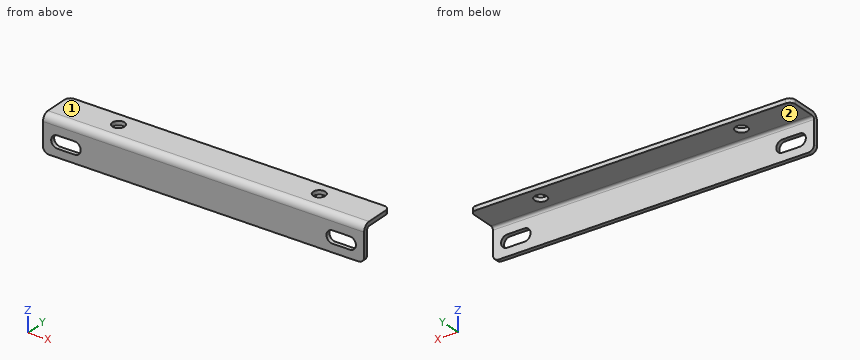
```python
from build123d import *

# Parameters (mm, degrees)
EXTRUDE1_DEPTH             = 88.9
FILLET1_R                  = 3.18
EXTRUDE2_REACH             = 94.271
EXTRUDE3_REACH             = 93.995
SKETCH3_R                  = 3.4036
FLATTEN_BENDS1_START       = -1.524
FLATTEN_BENDS1_OUTLINE_W   = 177.8
FLATTEN_BENDS1_OUTLINE_H   = 5.286
FLATTEN_BENDS1_DEPTH       = 17.4498
FLATTEN_BENDS1_START_2     = -3.81
FLATTEN_BENDS1_2_OUTLINE_R = 3.4036
FLATTEN_BENDS1_2_DEPTH     = 2.286
PROCESS_BENDS1_START       = 2.234903703
PROCESS_BENDS1_OUTLINE_W   = 177.8
PROCESS_BENDS1_OUTLINE_H   = 2.286
PROCESS_BENDS1_DEPTH       = 16.356210101
PROCESS_BENDS1_2_OUTLINE_R = 3.4036
PROCESS_BENDS1_2_DEPTH     = 1.8835878
PROCESS_BENDS1_START_2     = 2.04455268
PROCESS_BENDS1_3_OUTLINE_W = 177.8
PROCESS_BENDS1_3_OUTLINE_H = 2.286
PROCESS_BENDS1_3_DEPTH     = 0.190351023
PROCESS_BENDS1_START_3     = -1.524
PROCESS_BENDS1_4_OUTLINE_R = 3.4036
PROCESS_BENDS1_4_DEPTH     = 3.81
PROCESS_BENDS1_START_4     = -88.9
PROCESS_BENDS1_5_DEPTH     = 177.8


with BuildPart() as part:
    # Sketch1 → Extrude1 (new, symmetric)
    with BuildSketch(Plane(origin=(0, 0, 0), x_dir=(0, 0, -1), z_dir=(1, 0, 0))):
        with BuildLine():
            Line((17.5006, -3.81), (17.5006, -1.524))
            Line((17.5006, -1.524), (1.524, -1.524))
            ThreePointArc((1.524, -1.524), (0.446369265, -1.077630735), (0, 0))
            Line((0, 0), (0, 15.9258))
            Line((0, 15.9258), (-2.286, 15.9258))
            Line((-2.286, 15.9258), (-2.286, 0))
            ThreePointArc((-2.286, 0), (-1.170076836, -2.694076836), (1.524, -3.81))
            Line((1.524, -3.81), (17.5006, -3.81))
        make_face()
    extrude(amount=EXTRUDE1_DEPTH, both=True)

    # Fillet1
    fillet1_edges = [part.edges().sort_by_distance(p)[0] for p in [
        (-88.9, -2.667, -17.5006),
        (88.9, 15.9258, 1.143),
        (88.9, -2.667, -17.5006),
        (-88.9, 15.9258, 1.143),
    ]]
    fillet(fillet1_edges, radius=FILLET1_R)

    # Sketch2 → Extrude2 (cut, up to next)
    with BuildSketch(Plane(origin=(0, -1.524, 0), x_dir=(1, 0, 0), z_dir=(0, 1, 0)), mode=Mode.PRIVATE) as extrude2_sk1:
        with BuildLine():
            Line((80.9625, 12.9667), (71.4375, 12.9667))
            ThreePointArc((71.4375, 12.9667), (68.0339, 9.5631), (71.4375, 6.1595))
            Line((71.4375, 6.1595), (80.9625, 6.1595))
            ThreePointArc((80.9625, 6.1595), (84.3661, 9.5631), (80.9625, 12.9667))
        make_face()
    extrude2_tool1 = extrude(extrude2_sk1.sketch, amount=-EXTRUDE2_REACH, mode=Mode.PRIVATE) & part.part
    # Sketch2 → Extrude2 (cut, up to next)
    with BuildSketch(Plane(origin=(0, -1.524, 0), x_dir=(1, 0, 0), z_dir=(0, 1, 0)), mode=Mode.PRIVATE) as extrude2_sk2:
        with BuildLine():
            Line((-71.4375, 6.1595), (-80.9625, 6.1595))
            ThreePointArc((-80.9625, 6.1595), (-84.3661, 9.5631), (-80.9625, 12.9667))
            Line((-80.9625, 12.9667), (-71.4375, 12.9667))
            ThreePointArc((-71.4375, 12.9667), (-68.0339, 9.5631), (-71.4375, 6.1595))
        make_face()
    extrude2_tool2 = extrude(extrude2_sk2.sketch, amount=-EXTRUDE2_REACH, mode=Mode.PRIVATE) & part.part
    add(extrude2_tool1.solids().sort_by_distance((76.2, -1.524, -9.5631))[0], mode=Mode.SUBTRACT)
    add(extrude2_tool2.solids().sort_by_distance((-76.2, -1.524, -9.5631))[0], mode=Mode.SUBTRACT)

    # Sketch3 → Extrude3 (cut, up to next)
    with BuildSketch(Plane(origin=(0, 0, 0), x_dir=(-1, 0, 0), z_dir=(0, 0, -1)), mode=Mode.PRIVATE) as extrude3_sk1:
        with Locations(Location((-55.5625, 8.001, 0), (0, 0, 90))):
            Circle(SKETCH3_R)
    extrude3_tool1 = extrude(extrude3_sk1.sketch, amount=-EXTRUDE3_REACH, mode=Mode.PRIVATE) & part.part
    # Sketch3 → Extrude3 (cut, up to next)
    with BuildSketch(Plane(origin=(0, 0, 0), x_dir=(-1, 0, 0), z_dir=(0, 0, -1)), mode=Mode.PRIVATE) as extrude3_sk2:
        with Locations(Location((55.5625, 8.001, 0), (0, 0, 90))):
            Circle(SKETCH3_R)
    extrude3_tool2 = extrude(extrude3_sk2.sketch, amount=-EXTRUDE3_REACH, mode=Mode.PRIVATE) & part.part
    add(extrude3_tool1.solids().sort_by_distance((55.5625, 8.001, 0))[0], mode=Mode.SUBTRACT)
    add(extrude3_tool2.solids().sort_by_distance((-55.5625, 8.001, 0))[0], mode=Mode.SUBTRACT)

    # Flatten-Bends1: read off the stored shape, not the designer's step
    # Flatten-Bends1 outline → Flatten-Bends1 (cut)
    with BuildSketch(Plane(origin=(0, 0, 0), x_dir=(1, 0, 0), z_dir=(0, 1, 0)).offset(FLATTEN_BENDS1_START)):
        with Locations((0, 0.357)):
            Rectangle(FLATTEN_BENDS1_OUTLINE_W, FLATTEN_BENDS1_OUTLINE_H)
    extrude(amount=FLATTEN_BENDS1_DEPTH, mode=Mode.SUBTRACT)

    # Flatten-Bends1 2 outline → Flatten-Bends1 2 (add)
    with BuildSketch(Plane(origin=(0, 0, 0), x_dir=(1, 0, 0), z_dir=(0, 1, 0)).offset(FLATTEN_BENDS1_START_2)):
        with BuildLine():
            ThreePointArc((-88.9, -15.411113804), (-87.968599564, -17.659713368), (-85.72, -18.591113804))
            Line((-85.72, -18.591113804), (85.72, -18.591113804))
            ThreePointArc((85.72, -18.591113804), (87.968599564, -17.659713368), (88.9, -15.411113804))
            Line((88.9, -15.411113804), (88.9, 3))
            Line((88.9, 3), (-88.9, 3))
            Line((-88.9, 3), (-88.9, -15.411113804))
        make_face()
        with Locations((-55.5625, -10.666313804)):
            Circle(FLATTEN_BENDS1_2_OUTLINE_R, mode=Mode.SUBTRACT)
        with Locations((55.5625, -10.666313804)):
            Circle(FLATTEN_BENDS1_2_OUTLINE_R, mode=Mode.SUBTRACT)
    extrude(amount=FLATTEN_BENDS1_2_DEPTH)

    # Process-Bends1: read off the stored shape, not the designer's step
    # Process-Bends1 outline → Process-Bends1 (cut)
    with BuildSketch(Plane.XY.offset(PROCESS_BENDS1_START)):
        with Locations((0, -2.667)):
            Rectangle(PROCESS_BENDS1_OUTLINE_W, PROCESS_BENDS1_OUTLINE_H)
    extrude(amount=PROCESS_BENDS1_DEPTH, mode=Mode.SUBTRACT)

    # Process-Bends1 2 outline → Process-Bends1 2 (add)
    with BuildSketch(Plane.XY):
        with BuildLine():
            Line((-88.9, 12.7458), (-88.9, -1.524))
            Line((-88.9, -1.524), (88.9, -1.524))
            Line((88.9, -1.524), (88.9, 12.7458))
            ThreePointArc((88.9, 12.7458), (87.968599564, 14.994399564), (85.72, 15.9258))
            Line((85.72, 15.9258), (-85.72, 15.9258))
            ThreePointArc((-85.72, 15.9258), (-87.968599564, 14.994399564), (-88.9, 12.7458))
        make_face()
        with Locations((-55.5625, 8.001)):
            Circle(PROCESS_BENDS1_2_OUTLINE_R, mode=Mode.SUBTRACT)
        with Locations((55.5625, 8.001)):
            Circle(PROCESS_BENDS1_2_OUTLINE_R, mode=Mode.SUBTRACT)
    extrude(amount=PROCESS_BENDS1_2_DEPTH)

    # Process-Bends1 3 outline → Process-Bends1 3 (cut)
    with BuildSketch(Plane.XY.offset(PROCESS_BENDS1_START_2)):
        with Locations((0, -2.667)):
            Rectangle(PROCESS_BENDS1_3_OUTLINE_W, PROCESS_BENDS1_3_OUTLINE_H)
    extrude(amount=PROCESS_BENDS1_3_DEPTH, mode=Mode.SUBTRACT)

    # Process-Bends1 4 outline → Process-Bends1 4 (add)
    with BuildSketch(Plane.XY.offset(PROCESS_BENDS1_START_3)):
        with BuildLine():
            Line((-88.9, 12.7458), (-88.9, -1.524))
            Line((-88.9, -1.524), (88.9, -1.524))
            Line((88.9, -1.524), (88.9, 12.7458))
            ThreePointArc((88.9, 12.7458), (87.968599564, 14.994399564), (85.72, 15.9258))
            Line((85.72, 15.9258), (-85.72, 15.9258))
            ThreePointArc((-85.72, 15.9258), (-87.968599564, 14.994399564), (-88.9, 12.7458))
        make_face()
        with Locations((-55.5625, 8.001)):
            Circle(PROCESS_BENDS1_4_OUTLINE_R, mode=Mode.SUBTRACT)
        with Locations((55.5625, 8.001)):
            Circle(PROCESS_BENDS1_4_OUTLINE_R, mode=Mode.SUBTRACT)
    extrude(amount=PROCESS_BENDS1_4_DEPTH)

    # Process-Bends1 5 outline → Process-Bends1 5 (cut)
    with BuildSketch(Plane.YZ.offset(PROCESS_BENDS1_START_4)):
        with BuildLine():
            Line((15.9258, -1.524), (15.9258, 0))
            Line((15.9258, 0), (0, 0))
            ThreePointArc((0, 0), (-1.077630735, -0.446369265), (-1.524, -1.524))
            Line((-1.524, -1.524), (15.9258, -1.524))
        make_face()
        with BuildLine():
            ThreePointArc((-3.81, -1.524), (-2.694076836, 1.170076836), (0, 2.286))
            Line((0, 2.286), (-1.524, 2.286))
            Line((-1.524, 2.286), (-1.524, 2.04455268))
            Line((-1.524, 2.04455268), (-3.81, 2.04455268))
            Line((-3.81, 2.04455268), (-3.81, -1.524))
        make_face()
    extrude(amount=PROCESS_BENDS1_5_DEPTH, mode=Mode.SUBTRACT)


solid = part.part
```
Design review of the part built by this model. Coordinates are the model's own, in mm. Face numbers are marked on the shaded views. A direction names the side the tool comes from. Give positions to 0.01 mm unless a question says otherwise; leave off trailing zeros. Write each loop counter-clockwise with the first axis right and the second up, starting at its lowest first coordinate (ties: lowest second). Pieces come first, ordered by that corner, then holes. Notation, with made-up numbers: (-4.5, 0) - (53.5, 0) arc R22 ccw to (53.5, 13) - close; hole circle Ø8 at (63, -34.5). An arc over 180 degrees is marked (long way). Return JSON: item names as keys, results as strings. Group by question number.
(1) Machinability: for the marked faces 1 and 2, which of the approach directions +Z, -Z, +X, -X, +Y, -Y give a long, thin tool a straight path to every point of the face, cutting with its end or side? Answer none if there is none.
(2) We need section A-A, the plane z = -9.5. Give the boundary of the cut face in (x, y), then the cut area to 3 significant figures.
(3) Insertion check: pin 1 (4 mm diameter, centred on x = 14.5, y = 8, fed in from -Z); pin 2 (0.7 mm diameter, centred on x = 75, y = -2.5, fed in from +Z); pin 3 (1.8 mm diameter, centred on x = -75, y = -3, fed in from +Z) (3 decimals). Each pin has a flat end and moves straight along its axis. Give the tip position at first contact, or say it passes through.
(4) We need section B-B, the plane x = 8. Give the boundary of the cut face in (y, z), then the cut area to 3 significant figures.
(5) We need section C-C, the plane y = 1.5. Give the boundary of the cut face in (x, z).
(6) To check wall thickness, follow probe 1 along Z at (x, y) = (58.5, 6); probe 2 along Y at (x, z) = (-22.5, -14); probe 3 along Z at (x, y) = (77, -3). State the ranges of each line that lie inside material, in increasing order.
Reported:
{
 "1": {"face 1": "+Z, +X, -X, +Y, -Y", "face 2": "-Z, +X, -X, +Y"},
 "2": {"outline": "(-88.9, -3.81) - (-84.37, -3.81) - (-84.37, -1.52) - (-88.9, -1.52) - close; (-68.03, -3.81) - (68.03, -3.81) - (68.03, -1.52) - (-68.03, -1.52) - close; (84.37, -3.81) - (88.9, -3.81) - (88.9, -1.52) - (84.37, -1.52) - close", "area": "332 mm2"},
 "3": {"pin 1": "stops at z = 0", "pin 2": "stops at z = 1.62", "pin 3": "stops at z = 1.655"},
 "4": {"outline": "(-3.81, -17.5) - (-1.52, -17.5) - (-1.52, -1.52) arc R1.52 cw to (0, 0) - (15.93, 0) - (15.93, 2.29) - (0, 2.29) arc R3.81 ccw to (-3.81, -1.52) - close", "area": "82.5 mm2"},
 "5": {"outline": "(-88.9, 0) - (88.9, 0) - (88.9, 2.29) - (-88.9, 2.29) - close"},
 "6": {"probe 1": "z = 0 to 2.29", "probe 2": "y = -3.81 to -1.52", "probe 3": "z = -17.5 to -12.97, -6.16 to 0.82"}
}
